The listing builds one solid part. Answer for the finished solid, in the listing's coordinates (mm). Face numbers are marked on the shaded views. A direction names the side the tool comes from. Give positions to 0.01 mm unless a question says otherwise; leave off trailing zeros. Write each loop counter-clockwise with the first axis right and the second up, starting at its lowest first coordinate (ties: lowest second). Pieces come first, ordered by that corner, then holes.
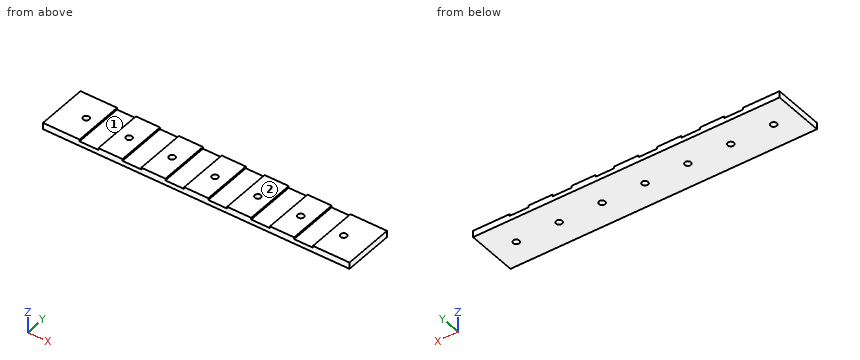
```python
from build123d import *

# Parameters (mm, degrees)
F0_W     = 150
F0_H     = 25
F1_DEPTH = 3.175
F2_W     = 9.2
F2_H     = 25
F3_DEPTH = 0.9
F4_R     = 1.5
F5_DEPTH = 25


with BuildPart() as f1:
    # F0 (on Top) → F1 (new body)
    with BuildSketch(Plane.XY):
        with Locations((75, 12.5)):
            Rectangle(F0_W, F0_H)
    extrude(amount=F1_DEPTH)

    # F2 (on face) → F3 (cut)
    with BuildSketch(Plane.XY.offset(3.175)):
        with Locations((22.5, 12.5)):
            Rectangle(F2_W, F2_H)
        with Locations((43.5, 12.5)):
            Rectangle(F2_W, F2_H)
        with Locations((64.5, 12.5)):
            Rectangle(F2_W, F2_H)
        with Locations((85.5, 12.5)):
            Rectangle(F2_W, F2_H)
        with Locations((106.5, 12.5)):
            Rectangle(F2_W, F2_H)
        with Locations((127.5, 12.5)):
            Rectangle(F2_W, F2_H)
    extrude(amount=-F3_DEPTH, mode=Mode.SUBTRACT)

    # F4 (on face) → F5 (cut)
    with BuildSketch(Plane.XY.offset(3.175)):
        with Locations((12, 12.5)):
            Circle(F4_R)
        with Locations((33, 12.5)):
            Circle(F4_R)
        with Locations((54, 12.5)):
            Circle(F4_R)
        with Locations((75, 12.5)):
            Circle(F4_R)
        with Locations((96, 12.5)):
            Circle(F4_R)
        with Locations((117, 12.5)):
            Circle(F4_R)
        with Locations((138, 12.5)):
            Circle(F4_R)
    extrude(amount=-F5_DEPTH, mode=Mode.SUBTRACT)


solid = f1.part
```
Item 1: A cutting plane is placed at B-B, the plane y = 6.5. Give the vertices of the cut face in (x, z) (3 decimals).
Conclusion:
outline: (0, 0) - (150, 0) - (150, 3.175) - (132.1, 3.175) - (132.1, 2.275) - (122.9, 2.275) - (122.9, 3.175) - (111.1, 3.175) - (111.1, 2.275) - (101.9, 2.275) - (101.9, 3.175) - (90.1, 3.175) - (90.1, 2.275) - (80.9, 2.275) - (80.9, 3.175) - (69.1, 3.175) - (69.1, 2.275) - (59.9, 2.275) - (59.9, 3.175) - (48.1, 3.175) - (48.1, 2.275) - (38.9, 2.275) - (38.9, 3.175) - (27.1, 3.175) - (27.1, 2.275) - (17.9, 2.275) - (17.9, 3.175) - (0, 3.175) - close
Item 2: A cutting plane is placed at C-C, the plane y = 12.5. Count the separate pieces of the cut face and the enclosed holes in it, plus the area to 3 significant figures.
Conclusion:
separate pieces: 8
enclosed holes: 0
area: 360 mm2
Item 3: A cutting plane is placed at A-A, the plane x = 33. Give the vertices of the cut face in (y, z) (3 decimals).
Conclusion:
outline: (0, 0) - (11, 0) - (11, 3.175) - (0, 3.175) - close; (14, 0) - (25, 0) - (25, 3.175) - (14, 3.175) - close
Item 4: Consider probe 1 along Y at (x, z) = (75, 1.35); probe 2 along Z at (x, y) = (44.5, 13) (3 decimals). Determine where each line is inside the solid, lowest interval first.
Conclusion:
probe 1: y = 0 to 11, 14 to 25
probe 2: z = 0 to 2.275
Item 5: Which of the six approach directions +Z, -Z, +X, -X, +Y, -Y give full straight-line access (tool end or side, diameter ignored) to the marked faces 1 and 2?
Conclusion:
face 1: +Z, +Y, -Y
face 2: +Z, +X, -X, +Y, -Y
Item 6: Each of these flat-tipped pins is pushed along its axis until it touches: P1, Ø2.5, axis at x = 96, y = 12.5, coming from the +Z side; P2, Ø3, axis at x = 22.5, y = 13, coming from the +Z side (3 decimals). Where does it stop, or does it pass through?
Conclusion:
P1: passes through
P2: stops at z = 2.275
